from build123d import *

# Parameters (mm, degrees)
BOX011_W       = 10
BOX011_H       = 10
BOX011_DEPTH   = 10
BOX012_W       = 10
BOX012_H       = 10
BOX012_DEPTH   = 10
BOX001_W       = 10
BOX001_H       = 10
BOX001_DEPTH   = 10
BOX003_W       = 10
BOX003_H       = 10
BOX003_DEPTH   = 10
BOX020_W       = 10
BOX020_H       = 10
BOX020_DEPTH   = 10
BOX019_W       = 10
BOX019_H       = 10
BOX019_DEPTH   = 10
BOX024_W       = 10
BOX024_H       = 10
BOX024_DEPTH   = 10
BOX017_W       = 10
BOX017_H       = 10
BOX017_DEPTH   = 10
BOX007_W       = 10
BOX007_H       = 10
BOX007_DEPTH   = 10
BOX013_W       = 10
BOX013_H       = 10
BOX013_DEPTH   = 10
BOX006_W       = 10
BOX006_H       = 10
BOX006_DEPTH   = 10
BOX005_W       = 10
BOX005_H       = 10
BOX005_DEPTH   = 10
BOX002_W       = 10
BOX002_H       = 10
BOX002_DEPTH   = 10
BOX015_W       = 10
BOX015_H       = 10
BOX015_DEPTH   = 10
BOX023_W       = 10
BOX023_H       = 10
BOX023_DEPTH   = 10
BOX004_W       = 10
BOX004_H       = 10
BOX004_DEPTH   = 10
BOX014_W       = 10
BOX014_H       = 10
BOX014_DEPTH   = 10
BOX009_W       = 10
BOX009_H       = 10
BOX009_DEPTH   = 10
BOX016_W       = 10
BOX016_H       = 10
BOX016_DEPTH   = 10
BOX010_W       = 10
BOX010_H       = 10
BOX010_DEPTH   = 10
BOX_W          = 10
BOX_H          = 10
BOX_DEPTH      = 10
BOX022_W       = 10
BOX022_H       = 10
BOX022_DEPTH   = 10
BOX018_W       = 10
BOX018_H       = 10
BOX018_DEPTH   = 10
BOX021_W       = 10
BOX021_H       = 10
BOX021_DEPTH   = 10
BOX008_W       = 10
BOX008_H       = 10
BOX008_DEPTH   = 10
CYLINDER_R     = 68
CYLINDER_DEPTH = 4


with BuildPart() as cubo011:
    # Box011 → Box011 (new body)
    with BuildSketch(Plane(origin=(-25, -5, 0), x_dir=(1, 0, 0), z_dir=(0, 0, 1))):
        with Locations((5, 5)):
            Rectangle(BOX011_W, BOX011_H)
    extrude(amount=BOX011_DEPTH)


with BuildPart() as cubo012:
    # Box012 → Box012 (new body)
    with BuildSketch(Plane(origin=(-15, -5, 0), x_dir=(1, 0, 0), z_dir=(0, 0, 1))):
        with Locations((5, 5)):
            Rectangle(BOX012_W, BOX012_H)
    extrude(amount=BOX012_DEPTH)


with BuildPart() as cubo001:
    # Box001 → Box001 (new body)
    with BuildSketch(Plane(origin=(-34.6, 34.5, 0), x_dir=(1, 0, 0), z_dir=(0, 0, 1))):
        with Locations((5, 5)):
            Rectangle(BOX001_W, BOX001_H)
    extrude(amount=BOX001_DEPTH)


with BuildPart() as cubo003:
    # Box003 → Box003 (new body)
    with BuildSketch(Plane(origin=(-25, 15, 0), x_dir=(1, 0, 0), z_dir=(0, 0, 1))):
        with Locations((5, 5)):
            Rectangle(BOX003_W, BOX003_H)
    extrude(amount=BOX003_DEPTH)


with BuildPart() as cubo020:
    # Box020 → Box020 (new body)
    with BuildSketch(Plane(origin=(-15.4, -34.6, 0), x_dir=(1, 0, 0), z_dir=(0, 0, 1))):
        with Locations((5, 5)):
            Rectangle(BOX020_W, BOX020_H)
    extrude(amount=BOX020_DEPTH)


with BuildPart() as cubo019:
    # Box019 → Box019 (new body)
    with BuildSketch(Plane(origin=(-25.4, -34.6, 0), x_dir=(1, 0, 0), z_dir=(0, 0, 1))):
        with Locations((5, 5)):
            Rectangle(BOX019_W, BOX019_H)
    extrude(amount=BOX019_DEPTH)


with BuildPart() as cubo024:
    # Box024 → Box024 (new body)
    with BuildSketch(Plane(origin=(-5, -15, 0), x_dir=(1, 0, 0), z_dir=(0, 0, 1))):
        with Locations((5, 5)):
            Rectangle(BOX024_W, BOX024_H)
    extrude(amount=BOX024_DEPTH)


with BuildPart() as cubo017:
    # Box017 → Box017 (new body)
    with BuildSketch(Plane(origin=(-25, -15, 0), x_dir=(1, 0, 0), z_dir=(0, 0, 1))):
        with Locations((5, 5)):
            Rectangle(BOX017_W, BOX017_H)
    extrude(amount=BOX017_DEPTH)


with BuildPart() as cubo007:
    # Box007 → Box007 (new body)
    with BuildSketch(Plane(origin=(-15, 5, 0), x_dir=(1, 0, 0), z_dir=(0, 0, 1))):
        with Locations((5, 5)):
            Rectangle(BOX007_W, BOX007_H)
    extrude(amount=BOX007_DEPTH)


with BuildPart() as cubo013:
    # Box013 → Box013 (new body)
    with BuildSketch(Plane(origin=(-55, -15, 0), x_dir=(1, 0, 0), z_dir=(0, 0, 1))):
        with Locations((5, 5)):
            Rectangle(BOX013_W, BOX013_H)
    extrude(amount=BOX013_DEPTH)


with BuildPart() as cubo006:
    # Box006 → Box006 (new body)
    with BuildSketch(Plane(origin=(-35, 5, 0), x_dir=(1, 0, 0), z_dir=(0, 0, 1))):
        with Locations((5, 5)):
            Rectangle(BOX006_W, BOX006_H)
    extrude(amount=BOX006_DEPTH)


with BuildPart() as cubo005:
    # Box005 → Box005 (new body)
    with BuildSketch(Plane(origin=(-45, 5, 0), x_dir=(1, 0, 0), z_dir=(0, 0, 1))):
        with Locations((5, 5)):
            Rectangle(BOX005_W, BOX005_H)
    extrude(amount=BOX005_DEPTH)


with BuildPart() as cubo002:
    # Box002 → Box002 (new body)
    with BuildSketch(Plane(origin=(-25, 25, 0), x_dir=(1, 0, 0), z_dir=(0, 0, 1))):
        with Locations((5, 5)):
            Rectangle(BOX002_W, BOX002_H)
    extrude(amount=BOX002_DEPTH)


with BuildPart() as cubo015:
    # Box015 → Box015 (new body)
    with BuildSketch(Plane(origin=(-35, -15, 0), x_dir=(1, 0, 0), z_dir=(0, 0, 1))):
        with Locations((5, 5)):
            Rectangle(BOX015_W, BOX015_H)
    extrude(amount=BOX015_DEPTH)


with BuildPart() as cubo023:
    # Box023 → Box023 (new body)
    with BuildSketch(Plane(origin=(-5, -5, 0), x_dir=(1, 0, 0), z_dir=(0, 0, 1))):
        with Locations((5, 5)):
            Rectangle(BOX023_W, BOX023_H)
    extrude(amount=BOX023_DEPTH)


with BuildPart() as cubo004:
    # Box004 → Box004 (new body)
    with BuildSketch(Plane(origin=(-15, 15, 0), x_dir=(1, 0, 0), z_dir=(0, 0, 1))):
        with Locations((5, 5)):
            Rectangle(BOX004_W, BOX004_H)
    extrude(amount=BOX004_DEPTH)


with BuildPart() as cubo014:
    # Box014 → Box014 (new body)
    with BuildSketch(Plane(origin=(-55, -25, 0), x_dir=(1, 0, 0), z_dir=(0, 0, 1))):
        with Locations((5, 5)):
            Rectangle(BOX014_W, BOX014_H)
    extrude(amount=BOX014_DEPTH)


with BuildPart() as cubo009:
    # Box009 → Box009 (new body)
    with BuildSketch(Plane(origin=(-45, -5, 0), x_dir=(1, 0, 0), z_dir=(0, 0, 1))):
        with Locations((5, 5)):
            Rectangle(BOX009_W, BOX009_H)
    extrude(amount=BOX009_DEPTH)


with BuildPart() as cubo016:
    # Box016 → Box016 (new body)
    with BuildSketch(Plane(origin=(-35, -25, 0), x_dir=(1, 0, 0), z_dir=(0, 0, 1))):
        with Locations((5, 5)):
            Rectangle(BOX016_W, BOX016_H)
    extrude(amount=BOX016_DEPTH)


with BuildPart() as cubo010:
    # Box010 → Box010 (new body)
    with BuildSketch(Plane(origin=(-35, -5, 0), x_dir=(1, 0, 0), z_dir=(0, 0, 1))):
        with Locations((5, 5)):
            Rectangle(BOX010_W, BOX010_H)
    extrude(amount=BOX010_DEPTH)


with BuildPart() as cubo:
    # Box → Box (new body)
    with BuildSketch(Plane(origin=(-35, 15, 0), x_dir=(1, 0, 0), z_dir=(0, 0, 1))):
        with Locations((5, 5)):
            Rectangle(BOX_W, BOX_H)
    extrude(amount=BOX_DEPTH)


with BuildPart() as cubo022:
    # Box022 → Box022 (new body)
    with BuildSketch(Plane(origin=(-5, 5, 0), x_dir=(1, 0, 0), z_dir=(0, 0, 1))):
        with Locations((5, 5)):
            Rectangle(BOX022_W, BOX022_H)
    extrude(amount=BOX022_DEPTH)


with BuildPart() as cubo018:
    # Box018 → Box018 (new body)
    with BuildSketch(Plane(origin=(-15, -15, 0), x_dir=(1, 0, 0), z_dir=(0, 0, 1))):
        with Locations((5, 5)):
            Rectangle(BOX018_W, BOX018_H)
    extrude(amount=BOX018_DEPTH)


with BuildPart() as cubo021:
    # Box021 → Box021 (new body)
    with BuildSketch(Plane(origin=(-5, 15, 0), x_dir=(1, 0, 0), z_dir=(0, 0, 1))):
        with Locations((5, 5)):
            Rectangle(BOX021_W, BOX021_H)
    extrude(amount=BOX021_DEPTH)


with BuildPart() as obj1:
    # Box008 → Box008 (new body)
    with BuildSketch(Plane(origin=(-55, -5, 0), x_dir=(1, 0, 0), z_dir=(0, 0, 1))):
        with Locations((5, 5)):
            Rectangle(BOX008_W, BOX008_H)
    extrude(amount=BOX008_DEPTH)

    # Fusion: union Cubo011, Cubo012, Cubo001, Cubo003, Cubo020, Cubo019, Cubo024, Cubo017, Cubo007, Cubo013, Cubo006, Cubo005, Cubo002, Cubo015, Cubo023, Cubo004, Cubo014, Cubo009, Cubo016, Cubo010, Cubo, Cubo022, Cubo018, Cubo021
    add(cubo011.part)
    add(cubo012.part)
    add(cubo001.part)
    add(cubo003.part)
    add(cubo020.part)
    add(cubo019.part)
    add(cubo024.part)
    add(cubo017.part)
    add(cubo007.part)
    add(cubo013.part)
    add(cubo006.part)
    add(cubo005.part)
    add(cubo002.part)
    add(cubo015.part)
    add(cubo023.part)
    add(cubo004.part)
    add(cubo014.part)
    add(cubo009.part)
    add(cubo016.part)
    add(cubo010.part)
    add(cubo.part)
    add(cubo022.part)
    add(cubo018.part)
    add(cubo021.part)


with BuildPart() as invaders:
    # Part__Mirroring: instance of obj1
    add(obj1.part.mirror(Plane(origin=(0, 0, 0), x_dir=(0, -1, 0), z_dir=(1, 0, 0))))

    # Fusion001: union obj1
    add(obj1.part)


with BuildPart() as invaders_final:
    # Cylinder → Cylinder (new body)
    with BuildSketch(Plane.XY.offset(-1)):
        Circle(CYLINDER_R)
    extrude(amount=CYLINDER_DEPTH)

    # Fusion002: union Invaders
    add(invaders.part)


solid = invaders_final.part
Geometry: final body of the model. Coordinates: model frame, mm. A direction names the side the tool comes from. Give positions to 0.01 mm unless a question says otherwise; leave off trailing zeros. Loops run counter-clockwise (first coordinate to the right, second up) from the corner with the lowest first, then second, coordinate; pieces in that order, holes last. Notation, with made-up numbers: (75.5, -4.5) -> (90.5, -4.5) arc R27 cw to (90.5, 13.5) -> close; hole circle Ø9 at (43.25, 73). An arc over 180 degrees is marked (long way). Put each result on its own line as item: value.
1. Pin query (flat end, axial travel): P1, Ø2, axis at y = -18.5, z = 8, coming from the +X side; P2, Ø2, axis at x = 49.5, z = 5.5, coming from the +Y side; P3, Ø2, axis at y = 40.5, z = 6.5, coming from the -X side. Return the tip coordinate at first contact, or that it passes through.
Taken from the geometry:
P1: stops at x = 55
P2: stops at y = 5
P3: stops at x = -34.6
2. Cut plane D-D (y = 42). Return the cut outline in (x, z).
Taken from the geometry:
outline: (-53.48, -1) -> (53.48, -1) -> (53.48, 3) -> (34.6, 3) -> (34.6, 10) -> (24.6, 10) -> (24.6, 3) -> (-24.6, 3) -> (-24.6, 10) -> (-34.6, 10) -> (-34.6, 3) -> (-53.48, 3) -> close
3. Set-up query: faces 1 (the flat face through (40, -5, 6)), 2 (the flat face through (-50, 5, 6)), 3 (the flat face through (15, 10, 6)), 4 (the flat face through (-25.4, -30, 6)). Return all of +Z, -Z, +X, -X, +Y, -Y with unobstructed straight access to the full face (end or side cutting, diameter ignored); none if empty.
Taken from the geometry:
face 1: +Z, -Y
face 2: +Z, -X, +Y
face 3: +Z
face 4: +Z, -X, -Y
4. Cut plane B-B (x = 0). Return the cut outline in (y, z), plus the area to 3 significant figures.
Taken from the geometry:
outline: (-68, -1) -> (68, -1) -> (68, 3) -> (25, 3) -> (25, 10) -> (-15, 10) -> (-15, 3) -> (-68, 3) -> close
area: 824 mm2
5. Pull-direction query (X, two-part tool) for faces 5 (the flat face through (24.6, 40, 6)), 6 (the flat face through (55, -10, 6)), 7 (the flat face through (-30, 34.5, 6)); classes: released by +X, released by -X, zero draft, split by the parting line, or undercut.
Taken from the geometry:
face 5: undercut
face 6: released by +X
face 7: zero draft
6. Cut plane C-C (z = 8). Count the separate pieces of the cut face and the enclosed holes in it, plus the area to 3 significant figures.
Taken from the geometry:
separate pieces: 1
enclosed holes: 2
area: 4,600 mm2
7. Ray query, line 1 along X through (y, z) = (-5.5, 9); line 2 along X through (y, z) = (14, 5.75); line 3 along Y through (x, z) = (-19, 8). Return the intervals inside material, ascending. Write a range as [from, to].
Taken from the geometry:
line 1: x = [-55, -45], [-35, 35], [45, 55]
line 2: x = [-45, -25], [-15, 15], [25, 45]
line 3: y = [-34.6, -24.6], [-15, 5], [15, 35]
8. Cut plane A-A (y = 0). Return the cut outline in (x, z), plus the area to 3 significant figures.
Taken from the geometry:
outline: (-68, -1) -> (68, -1) -> (68, 3) -> (55, 3) -> (55, 10) -> (-55, 10) -> (-55, 3) -> (-68, 3) -> close
area: 1,310 mm2
